from build123d import *

# Parameters (mm, degrees)
SKETCH1_W           = 96.2
SKETCH1_H           = 294.64
SKETCH1_R           = 1.3890625
SKETCH1_R_2         = 3.175
SKETCH1_R_3         = 9.7282
SKETCH1_W_2         = 6.35
SKETCH1_H_2         = 6.35
BOSS_EXTRUDE1_DEPTH = 6.35
SKETCH3_W           = 6.35
SKETCH3_H           = 294.64
CUT_EXTRUDE2_DEPTH  = 6.35
SKETCH4_W           = 6.35
SKETCH4_H           = 294.64
CUT_EXTRUDE3_DEPTH  = 6.35


with BuildPart() as part:
    # Sketch1 → Boss-Extrude1 (new body)
    with BuildSketch(Plane.XY):
        with Locations((48.1, 147.32)):
            Rectangle(SKETCH1_W, SKETCH1_H)
        with Locations((63.9749986, 120.65)):
            Circle(SKETCH1_R, mode=Mode.SUBTRACT)
        with Locations((63.9749986, 133.35)):
            Circle(SKETCH1_R_2, mode=Mode.SUBTRACT)
        with Locations((63.9749986, 146.05)):
            Circle(SKETCH1_R, mode=Mode.SUBTRACT)
        with Locations((32.2250014, 146.05)):
            Circle(SKETCH1_R, mode=Mode.SUBTRACT)
        with Locations((32.2250014, 133.35)):
            Circle(SKETCH1_R_2, mode=Mode.SUBTRACT)
        with Locations((32.2250014, 120.65)):
            Circle(SKETCH1_R, mode=Mode.SUBTRACT)
        with Locations((60.754989798, 179.209178053)):
            Circle(SKETCH1_R, mode=Mode.SUBTRACT)
        with Locations((26.464989798, 179.209178053)):
            Circle(SKETCH1_R, mode=Mode.SUBTRACT)
        with Locations((43.609989798, 179.209178053)):
            Circle(SKETCH1_R_3, mode=Mode.SUBTRACT)
        with Locations((86.2, 257.175)):
            Rectangle(SKETCH1_W_2, SKETCH1_H_2, mode=Mode.SUBTRACT)
        with Locations((76.675, 257.175)):
            Rectangle(SKETCH1_W_2, SKETCH1_H_2, mode=Mode.SUBTRACT)
        with Locations((19.525, 257.175)):
            Rectangle(SKETCH1_W_2, SKETCH1_H_2, mode=Mode.SUBTRACT)
        with Locations((10, 257.175)):
            Rectangle(SKETCH1_W_2, SKETCH1_H_2, mode=Mode.SUBTRACT)
    extrude(amount=BOSS_EXTRUDE1_DEPTH)

    # Sketch3 → Cut-Extrude2 (cut)
    with BuildSketch(Plane.ZY):
        with Locations((3.175, 147.32)):
            Rectangle(SKETCH3_W, SKETCH3_H)
    extrude(amount=-CUT_EXTRUDE2_DEPTH, mode=Mode.SUBTRACT)

    # Sketch4 → Cut-Extrude3 (cut)
    with BuildSketch(Plane(origin=(96.2, 0, 0), x_dir=(0, 0, -1), z_dir=(1, 0, 0))):
        with Locations((-3.175, 147.32)):
            Rectangle(SKETCH4_W, SKETCH4_H)
    extrude(amount=-CUT_EXTRUDE3_DEPTH, mode=Mode.SUBTRACT)


solid = part.part
Part model, mm, in its own coordinate system. A direction names the side the tool comes from. Coordinates: 2 decimals unless noted, no trailing zeros. Loops run counter-clockwise (first coordinate to the right, second up) from the corner with the lowest first, then second, coordinate; pieces in that order, holes last. Notation, with made-up numbers: (42.25, -28) -> (51.25, -28) arc R21 ccw to (51.25, 6) -> close; hole circle Ø4 at (20, 84). An arc over 180 degrees is marked (long way). Use a Markdown table: item, result. Add a question column.
Item 1: Flat gauge pin, fed straight in: P1, Ø3, axis at x = 84.5, z = 2.5, coming from the -Y side. Where does the tip first touch, or does it go through?
Item 2: Band-saw the part on A-A on y = 133.35. Write the cut outline in (x, z), plus the area to 3 significant figures.
Item 3: Probe probe 1 along Y at (x, z) = (32, 0.75); probe 2 along X at (y, z) = (146.05, 4.5); probe 3 along X at (y, z) = (133.35, 4.5). List the from-to ranges inside material, lowest first.
Item 4: Band-saw the part on B-B on x = 43. Write the cut outline in (y, z), plus the area to 3 significant figures.
Item 5: Pull direction Y, two halves, no side cores. Call faces 3 (the flat face through (48, 149, 6.35)), 4 (the flat face through (19, 254, 3)), 5 (the flat face through (48, 0, 3)): +Y half, -Y half, draft (parallel to the pull), parting line (faces both ways), or undercut.
Item 6: Which spindle directions (+Z, -Z, +X, -X, +Y, -Y) get a long thin tool onto all of the face, cutting with end or side? Do faces 1 (the flat face through (86, 254, 3)), 2 (the flat face through (48, 294.64, 3)). Say none if no direction does.
Item 7: Band-saw the part on C-C on z = 2.75. Give the number of separate pieces and of enclosed holes in the cut face, plus the area to 3 significant figures.
Geometry says:
| question | item | result |
|---|---|---|
| 1 | P1 | y = 0 |
| 2 | outline | (6.35, 0) -> (29.05, 0) -> (29.05, 6.35) -> (6.35, 6.35) -> close; (35.4, 0) -> (60.8, 0) -> (60.8, 6.35) -> (35.4, 6.35) -> close; (67.15, 0) -> (89.85, 0) -> (89.85, 6.35) -> (67.15, 6.35) -> close |
| 2 | area | 450 mm² |
| 3 | probe 1 | 0 to 119.28, 122.02 to 130.18, 136.52 to 144.68, 147.42 to 294.64 |
| 3 | probe 2 | 6.35 to 30.84, 33.61 to 62.59, 65.36 to 89.85 |
| 3 | probe 3 | 6.35 to 29.05, 35.4 to 60.8, 67.15 to 89.85 |
| 4 | outline | (0, 0) -> (169.5, 0) -> (169.5, 6.35) -> (0, 6.35) -> close; (188.92, 0) -> (294.64, 0) -> (294.64, 6.35) -> (188.92, 6.35) -> close |
| 4 | area | 1,750 mm² |
| 5 | face 3 | draft |
| 5 | face 4 | undercut |
| 5 | face 5 | -Y half |
| 6 | face 1 | +Z, -Z |
| 6 | face 2 | +Z, -Z, +X, -X, +Y |
| 7 | separate pieces | 1 |
| 7 | enclosed holes | 13 |
| 7 | area | 24,000 mm² |
